Could you check a few things on this drawing? It's one solid part, dimensions in mm from its lowest x, y, z. Coordinates: 2 decimals unless noted, no trailing zeros. Order: outer loops, then holes, each group sorted by start corner. A loop starts at its lowest first (then second) coordinate and runs counter-clockwise, first axis right, second up. Notation, with made-up numbers: (34, 61.5) -> (38, 61.5) arc R26 cw to (38, 94.5) -> close; hole circle Ø3 at (-35, 10). An arc over 180 degrees is marked (long way). Use a Markdown table: item, result. Add a question column.
1. Suppose I cut it at A-A, the plane z = 12.6. List the corners of the cut face in (x, y) for me, then the cut area to 3 significant figures.
2. Suppose I cut it at C-C, the plane x = 12.25. List the corners of the cut face in (y, z) for me.
3. Suppose I cut it at B-B, the plane y = 7. List the corners of the cut face in (x, z) for me (1 decimal), then the cut area to 3 significant figures.
4. For pin 1 Ø6.5 at (x, y) = (15, 7.5) entering from +Z; pin 2 Ø17 at (x, y) = (19, 14.5) entering from -Z; pin 3 Ø12 at (y, z) = (5.5, 6) entering from -X (1 decimal), each with a flat end and sliding along its axis, tell me the tip position at first contact or that it passes through.
5. We'd pull the mould along Y, two halves only. Please class the marked faces 1, 2 and 3: pulls with the +Y half, pulls with the -Y half, needs draft (parallel to the pull), parting line crosses it, or undercut.
6. If I drill on line 1 along Z through (x, y) = (11, 10.25); line 2 along Y through (x, z) = (25.5, 21.5); line 3 along Y through (x, z) = (23, 10) (1 decimal), over which ranges is the centre line in solid material (lowest first)? Write a range as from..to.
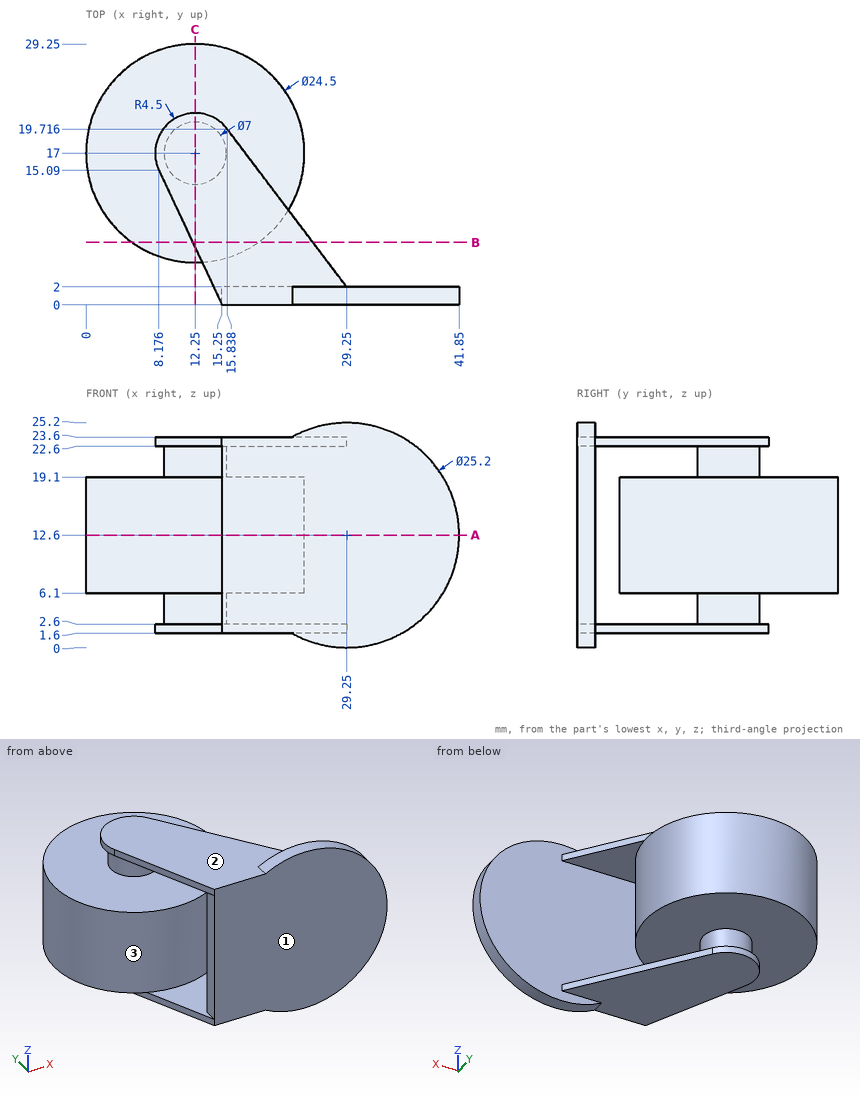
Worked out:
| question | item | result |
|---|---|---|
| 1 | outline | circle Ø24.5 at (12.25, 17); (15.25, 0) -> (41.85, 0) -> (41.85, 2) -> (15.25, 2) -> close |
| 1 | area | 525 mm² |
| 2 | outline | (4.75, 6.1) -> (13.5, 6.1) -> (13.5, 2.6) -> (6.4, 2.6) -> (6.4, 1.6) -> (21.5, 1.6) -> (21.5, 2.6) -> (20.5, 2.6) -> (20.5, 6.1) -> (29.25, 6.1) -> (29.25, 19.1) -> (20.5, 19.1) -> (20.5, 22.6) -> (21.5, 22.6) -> (21.5, 23.6) -> (6.4, 23.6) -> (6.4, 22.6) -> (13.5, 22.6) -> (13.5, 19.1) -> (4.75, 19.1) -> close |
| 3 | outline | (5.2, 6.1) -> (19.3, 6.1) -> (19.3, 19.1) -> (5.2, 19.1) -> close; (12, 1.6) -> (25.5, 1.6) -> (25.5, 2.6) -> (12, 2.6) -> close; (12, 22.6) -> (25.5, 22.6) -> (25.5, 23.6) -> (12, 23.6) -> close |
| 3 | area | 211 mm² |
| 4 | pin 1 | stops at z = 23.6 |
| 4 | pin 2 | stops at z = 1.6 |
| 4 | pin 3 | stops at x = 1.3 |
| 5 | face 1 | pulls with the -Y half |
| 5 | face 2 | needs draft |
| 5 | face 3 | undercut |
| 6 | line 1 | z = 1.6..2.6, 6.1..19.1, 22.6..23.6 |
| 6 | line 2 | y = 0..2 |
| 6 | line 3 | y = 0..2, 11.1..22.9 |
